from build123d import *

# Parameters (mm, degrees)
F1_DEPTH  = 70
F2_R      = 4
F3_DEPTH  = 10
F4_R      = 4
F5_DEPTH  = 10
F6_R      = 4
F7_DEPTH  = 10
F8_R      = 4
F9_DEPTH  = 10
F10_R     = 4
F11_DEPTH = 10


with BuildPart() as f1:
    # F0 (on Front) → F1 (new body)
    with BuildSketch(Plane.XZ):
        Polygon((0, 25.5), (-10, 15.5), (-10, -39.5), (10, -39.5), (10, 15.5), align=None)
    extrude(amount=F1_DEPTH)

    # F2 (on face) → F3 (cut)
    with BuildSketch(Plane.XZ.offset(70)):
        with Locations((0, -29.5)):
            Circle(F2_R)
    extrude(amount=-F3_DEPTH, mode=Mode.SUBTRACT)

    # F4 (on face) → F5 (cut)
    with BuildSketch(Plane.XZ.offset(70)):
        with Locations((0, 15.5)):
            Circle(F4_R)
    extrude(amount=-F5_DEPTH, mode=Mode.SUBTRACT)

    # F6 (on face) → F7 (cut)
    with BuildSketch(Plane(origin=(0, 0, 0), x_dir=(-1, 0, 0), z_dir=(0, 1, 0))):
        with Locations((0, -29.5)):
            Circle(F6_R)
    extrude(amount=-F7_DEPTH, mode=Mode.SUBTRACT)

    # F8 (on face) → F9 (cut)
    with BuildSketch(Plane(origin=(0, 0, 0), x_dir=(-1, 0, 0), z_dir=(0, 1, 0))):
        with Locations((0, 15.5)):
            Circle(F8_R)
    extrude(amount=-F9_DEPTH, mode=Mode.SUBTRACT)

    # F10 (on face) → F11 (cut)
    with BuildSketch(Plane(origin=(0, 0, -39.5), x_dir=(1, 0, 0), z_dir=(0, 0, -1))):
        with Locations((0, 35)):
            Circle(F10_R)
    extrude(amount=-F11_DEPTH, mode=Mode.SUBTRACT)


solid = f1.part
Verification items for the finished model (mm, model axes). A direction names the side the tool comes from. Coordinates: 2 decimals unless noted, no trailing zeros. Loops run counter-clockwise (first coordinate to the right, second up) from the corner with the lowest first, then second, coordinate; pieces in that order, holes last. Notation, with made-up numbers: (28.25, 60) -> (37.25, 60) arc R32 cw to (37.25, 99) -> close; hole circle Ø2 at (81, 56.25). An arc over 180 degrees is marked (long way). Answer as a JSON object with one key per item and string values. Group by question number.
Item 1: Tool access check on faces 1 (the flat face through (5.1, -34.5, 20.4)), 2 (the flat face through (0, -60, 16)), 3 (the flat face through (0, -35, -29.5)), 4 (the flat face through (0, -10, -29)), 5 (the flat face through (-4.9, -34.5, 20.6)). Record the directions out of +Z, -Z, +X, -X, +Y, -Y that give a thin tool (end or side, any length) a straight path to the whole face; none if there is none.
Item 2: Scan lines: probe 1 along Z at (x, y) = (0, -67.5); probe 2 along X at (y, z) = (-35, -32.5); probe 3 along Y at (x, z) = (-2.75, 17). Record each from-to range of solid material in increasing order.
Item 3: Sectioned sample at D-D on x = 2. Record the boundary of the cut face in (y, z).
Item 4: Depth check by flat-ended pin: pin 1 (10 mm diameter, centred on x = 6, y = -13.5, fed in from +Z); pin 2 (4 mm diameter, centred on x = -1.5, z = -30.5, fed in from +Y); pin 3 (2.5 mm diameter, centred on x = -0.5, z = -28, fed in from -Y). Enter the tip coordinate at first touch or a pass-through.
Item 5: Sectioned sample at B-B on z = -32. Record the boundary of the cut face in (x, y), plus the area to 3 significant figures.
Item 6: Mould release check, pull along X, two halves, no side actions. Record for faces 6 (the flat face through (10, -35, -12)), 7 (the flat face through (0, -10, 16)), 8 (the flat face through (0, 0, -7)): +X half, -X half, draft (parallel to the pull), parting line (faces both ways), or undercut.
Item 7: Sectioned sample at A-A on y = -63. Record the boundary of the cut face in (x, z), plus the area to 3 significant figures.
Item 8: Sectioned sample at C-C on y = -35. Record the boundary of the cut face in (x, z), plus the area to 3 significant figures.
Evaluation:
{
 "1": {"face 1": "+Z, +X, +Y, -Y", "face 2": "-Y", "face 3": "-Z", "face 4": "+Y", "face 5": "+Z, -X, +Y, -Y"},
 "2": {"probe 1": "z = -39.5 to -33.5, -25.5 to 11.5, 19.5 to 25.5", "probe 2": "x = -10 to -4, 4 to 10", "probe 3": "y = -60 to -10"},
 "3": {"outline": "(-70, -39.5) -> (-38.46, -39.5) -> (-38.46, -29.5) -> (-31.54, -29.5) -> (-31.54, -39.5) -> (0, -39.5) -> (0, -32.96) -> (-10, -32.96) -> (-10, -26.04) -> (0, -26.04) -> (0, 12.04) -> (-10, 12.04) -> (-10, 18.96) -> (0, 18.96) -> (0, 23.5) -> (-70, 23.5) -> (-70, 18.96) -> (-60, 18.96) -> (-60, 12.04) -> (-70, 12.04) -> (-70, -26.04) -> (-60, -26.04) -> (-60, -32.96) -> (-70, -32.96) -> close"},
 "4": {"pin 1": "stops at z = 24.5", "pin 2": "stops at y = -10", "pin 3": "stops at y = -60"},
 "5": {"outline": "(-10, -70) -> (-3.12, -70) -> (-3.12, -60) -> (3.12, -60) -> (3.12, -70) -> (10, -70) -> (10, 0) -> (3.12, 0) -> (3.12, -10) -> (-3.12, -10) -> (-3.12, 0) -> (-10, 0) -> close; hole circle Ø8 at (0, -35)", "area": "1,220 mm²"},
 "6": {"face 6": "+X half", "face 7": "undercut", "face 8": "draft"},
 "7": {"outline": "(-10, -39.5) -> (10, -39.5) -> (10, 15.5) -> (0, 25.5) -> (-10, 15.5) -> close; hole circle Ø8 at (0, -29.5); hole circle Ø8 at (0, 15.5)", "area": "1,100 mm²"},
 "8": {"outline": "(-10, -39.5) -> (-4, -39.5) -> (-4, -29.5) -> (4, -29.5) -> (4, -39.5) -> (10, -39.5) -> (10, 15.5) -> (0, 25.5) -> (-10, 15.5) -> close", "area": "1,120 mm²"}
}
